Could you check a few things on this model? Use its own coordinates, in mm. Give positions to 0.01 mm unless a question says otherwise; leave off trailing zeros. Loops run counter-clockwise (first coordinate to the right, second up) from the corner with the lowest first, then second, coordinate; pieces in that order, holes last. Notation, with made-up numbers: (11.5, -22) -> (54.5, -22) arc R16 cw to (54.5, 4) -> close; hole circle Ø11 at (10, 77.5). An arc over 180 degrees is marked (long way). Write each question's results on one line, items separated by ' | '. Start each with the question number.
Q1. If I drill on line 1 along Y through (x, z) = (0.5, 0.15); line 2 along X through (y, z) = (13.5, 0.25); line 3 along Y through (x, z) = (-2.5, 1.6), over which ranges is the centre line in solid material (lowest first)?
Q2. Will these pins go through, and if not, where does the flat tip stop? P1, Ø1, axis at x = 32, z = 1, coming from the -Y side; P2, Ø0.6, axis at x = -7.5, z = 1, coming from the -Y side; P3, Ø0.6, axis at y = -2.5, z = 1.5, coming from the -X side.
Q3. If we section it at C-C, the plane y = -200: List the corners of the cut face in (x, z) for me, plus the area to 3 significant figures.
Q4. We'd pull the mould along X, two halves only. Please class faces 1 (the face through (-11.15, -184.73, 0.99)), 2 (the face through (23.874, -194.787, 0.986)), 3 (the face through (-1.56, -188.1, 0.99)), 4 (the face through (14, -76, 2)): released by +X, released by -X, zero draft, split by the parting line, or undercut.
Q5. If we section it at A-A, the plane x = 20: List the corners of the cut face in (y, z) for me, plus the area to 3 significant figures.
Q6. If we section it at B-B, the plane z = 0.5: Give the number of separate pieces and of enclosed holes in the cut face, plus the area to 3 significant figures.
from build123d import *

# Parameters (mm, degrees)
SKETCH_1_R      = 12
SKETCH_1_W      = 32
SKETCH_1_H      = 2
SKETCH_1_W_2    = 25
SKETCH_1_H_2    = 60
EXTRUDE_1_DEPTH = 2


with BuildPart() as part:
    # 草图1 → 凸台-拉伸1 (new body)
    with BuildSketch(Plane.XY):
        with BuildLine():
            Line((-8, -48.342527861), (-6, -48.342527861))
            Line((-6, -48.342527861), (-6, -68.342527861))
            Line((-6, -68.342527861), (-8, -68.342527861))
            Line((-8, -68.342527861), (-8, -88.342527861))
            Line((-8, -88.342527861), (-6, -88.342527861))
            Line((-6, -88.342527861), (-6, -108.342527861))
            Line((-6, -108.342527861), (-8, -108.342527861))
            Line((-8, -108.342527861), (-8, -128.342527861))
            Line((-8, -128.342527861), (-6, -128.342527861))
            Line((-6, -128.342527861), (-6, -144.000000011))
            Line((-6, -144.000000011), (-8, -144.000000011))
            Line((-8, -144.000000011), (-8, -174))
            Line((-8, -174), (-14.392579, -195.774639692))
            ThreePointArc((-14.392579, -195.774639692), (-12.007922481, -208.989426995), (0, -215))
            Line((0, -215), (15, -215))
            Line((15, -215), (33, -174))
            Line((33, -174), (31, -174))
            Line((31, -174), (31, -156.221540553))
            Line((31, -156.221540553), (33, -156.221540553))
            Line((33, -156.221540553), (33, -136.221540553))
            Line((33, -136.221540553), (31, -136.221540553))
            Line((31, -136.221540553), (31, -116.221540553))
            Line((31, -116.221540553), (33, -116.221540553))
            Line((33, -116.221540553), (33, -96.221540553))
            Line((33, -96.221540553), (31, -96.221540553))
            Line((31, -96.221540553), (31, -76.221540553))
            Line((31, -76.221540553), (33, -76.221540553))
            Line((33, -76.221540553), (33, -56.221540553))
            Line((33, -56.221540553), (31, -56.221540553))
            Line((31, -56.221540553), (31, -36.221540553))
            Line((31, -36.221540553), (33, -36.221540553))
            Line((33, -36.221540553), (33, -16.221540553))
            Line((33, -16.221540553), (31, -16.221540553))
            Line((31, -16.221540553), (31, 3.778459447))
            Line((31, 3.778459447), (33, 3.778459447))
            Line((33, 3.778459447), (33, 23.778459447))
            Line((33, 23.778459447), (31, 23.778459447))
            Line((31, 23.778459447), (31, 43.778459447))
            Line((31, 43.778459447), (33, 43.778459447))
            Line((33, 43.778459447), (33, 49))
            Line((33, 49), (33, 59))
            Line((33, 59), (-6, 59))
            Line((-6, 59), (-6, 51.657472139))
            Line((-6, 51.657472139), (-8, 51.657472139))
            Line((-8, 51.657472139), (-8, 31.657472139))
            Line((-8, 31.657472139), (-6, 31.657472139))
            Line((-6, 31.657472139), (-6, 11.657472139))
            Line((-6, 11.657472139), (-8, 11.657472139))
            Line((-8, 11.657472139), (-8, -8.342527861))
            Line((-8, -8.342527861), (-6, -8.342527861))
            Line((-6, -8.342527861), (-6, -28.342527861))
            Line((-6, -28.342527861), (-8, -28.342527861))
            Line((-8, -28.342527861), (-8, -48.342527861))
        make_face()
        with Locations((0, -200)):
            Circle(SKETCH_1_R, mode=Mode.SUBTRACT)
        with Locations((12, -55.221540553)):
            Rectangle(SKETCH_1_W, SKETCH_1_H, mode=Mode.SUBTRACT)
        with Locations((12, -95.221540553)):
            Rectangle(SKETCH_1_W, SKETCH_1_H, mode=Mode.SUBTRACT)
        with Locations((12, -135.221540553)):
            Rectangle(SKETCH_1_W, SKETCH_1_H, mode=Mode.SUBTRACT)
        with Locations((12.5, 0)):
            Rectangle(SKETCH_1_W_2, SKETCH_1_H_2, mode=Mode.SUBTRACT)
    extrude(amount=EXTRUDE_1_DEPTH)


solid = part.part
Final values:
1) line 1: y = -215 to -211.99, -188.01 to -136.22, -134.22 to -96.22, -94.22 to -56.22, -54.22 to -30, 30 to 59 | line 2: x = -6 to 0, 25 to 33 | line 3: y = -214.79 to -211.74, -188.26 to -136.22, -134.22 to -96.22, -94.22 to -56.22, -54.22 to 59
2) P1: stops at y = -177.42 | P2: stops at y = -213.16 | P3: stops at x = -8
3) outline: (-15, 0) -> (-12, 0) -> (-12, 2) -> (-15, 2) -> close; (12, 0) -> (21.59, 0) -> (21.59, 2) -> (12, 2) -> close | area: 25.2 mm²
4) face 1: released by -X | face 2: released by +X | face 3: undercut | face 4: zero draft
5) outline: (-203.61, 0) -> (-136.22, 0) -> (-136.22, 2) -> (-203.61, 2) -> close; (-134.22, 0) -> (-96.22, 0) -> (-96.22, 2) -> (-134.22, 2) -> close; (-94.22, 0) -> (-56.22, 0) -> (-56.22, 2) -> (-94.22, 2) -> close; (-54.22, 0) -> (-30, 0) -> (-30, 2) -> (-54.22, 2) -> close; (30, 0) -> (59, 0) -> (59, 2) -> (30, 2) -> close | area: 393 mm²
6) separate pieces: 1 | enclosed holes: 5 | area: 8,430 mm²
